Autodesk Inventor part; units mm, degrees
ref_plane "YZ Plane" through (0, 0, 0) normal (1, 0, 0) x (0, 1, 0)
ref_plane "XZ Plane" through (0, 0, 0) normal (0, 1, 0) x (-1, 0, 0)
ref_plane "XY Plane" through (0, 0, 0) normal (0, 0, 1) x (1, 0, 0)
sketch "Sketch1" plane through (0, 0, 0) normal (0, 0, 1) x (1, 0, 0)
  line L0 (-127, 177.8) -> (127, 177.8)
  line L1 (127, 177.8) -> (127, -177.8)
  line L2 (127, -177.8) -> (-127, -177.8)
  line L3 (-127, -177.8) -> (-127, 177.8)
  point P0 (0, 0)
  dimension "d0" = 254
  dimension "d1" = 127
  dimension "d2" = 355.6
  dimension "d3" = 177.8
extrude "Extrusion1" add sketch "Sketch1" along normal blind 6.35
sketch "Sketch2" plane through (0, 0, 6.35) normal (0, 0, 1) x (1, 0, 0)
  line L0 (-114.3, 165.1) -> (114.3, 165.1) construction
  line L1 (114.3, 165.1) -> (114.3, -165.1) construction
  line L2 (114.3, -165.1) -> (-114.3, -165.1) construction
  line L3 (-114.3, -165.1) -> (-114.3, 165.1) construction
  line L4 (-127, 177.8) -> (127, 177.8) construction
  line L5 (127, -177.8) -> (-127, -177.8) construction
  line L6 (-127, -177.8) -> (-127, 177.8) construction
  line L7 (127, 177.8) -> (127, -177.8) construction
  point P0 (0, 0)
  point P1 (0, 0)
  dimension "d6" = 12.7
  dimension "d7" = 12.7
  dimension "d8" = 12.7
  dimension "d9" = 12.7
hole "Hole1" at (-114.3, 165.1, 6.35) at (114.3, 165.1, 6.35) at (114.3, -165.1, 6.35) at (-114.3, -165.1, 6.35) at (0, 0, 6.35) direction (0, 0, -1) diameter 6.7564 end through all
sketch "Sketch3" plane through (0, 0, 6.35) normal (0, 0, 1) x (1, 0, 0)
  line L0 (0, 248.92) -> (0, -248.92) construction
  point P0 (0, 0)
  point P1 (0, 119.38)
  point P2 (0, -119.38)
  dimension "d17" = 238.76
  dimension "d18" = 119.38
hole "Hole2" at (0, 119.38, 6.35) at (0, -119.38, 6.35) direction (0, 0, -1) diameter 44.45 end through all
sketch "Sketch4" plane through (0, 0, 6.35) normal (0, 0, 1) x (1, 0, 0)
  line L0 (0, -248.92) -> (0, 248.92) construction
  circle A0 centre (0, 119.38) radius 22.225 construction
  circle A1 centre (0, -119.38) radius 22.225 construction
  line L1 (-177.8, 0) -> (177.8, 0) construction
  point P0 (0, 0)
  point P1 (0, 68.58)
  point P2 (0, 43.18)
  point P3 (0, -68.58)
  point P4 (0, -43.18)
  dimension "d26" = 50.8
  dimension "d27" = 25.4
  dimension "d28" = 50.8
  dimension "d29" = 25.4
hole "Hole3" at (0, 68.58, 6.35) at (0, 43.18, 6.35) at (0, -68.58, 6.35) at (0, -43.18, 6.35) direction (0, 0, -1) diameter 3.302 end through all
fillet "Fillet1" radius 12.7 4 edges at (127, -177.8, 3.175) (-127, -177.8, 3.175) (127, 177.8, 3.175) (-127, 177.8, 3.175)
chamfer "Chamfer1" distance 3.175 angle 45 2 edges at (0, -97.155, 6.35) (0, 141.605, 6.35)
sketch "Sketch6" plane through (127, -165.1, 0) normal (1, 0, 0) x (0, 0, -1)
  line L0 (-6.35, 330.2) -> (0, 330.2)
  line L1 (-6.35, 330.2) -> (-6.35, 0)
  line L2 (0, 0) -> (-6.35, 0)
  line L3 (0, 330.2) -> (0, 0)
  line L4 (-3.175, 330.2) -> (-3.175, 0) construction
  line L5 (0, 165.1) -> (-6.35, 165.1) construction
  point P0 (-3.175, 165.1)
  point P1 (-3.175, 311.15)
  point P2 (-3.175, 19.05)
  dimension "d52" = 146.05
hole "Hole5" at (127, 0, 3.175) at (127, 146.05, 3.175) at (127, -146.05, 3.175) direction (-1, 0, 0) diameter 2.6416 depth 15.24 tip angle 118
mirror "Mirror1" about plane through (0, 0, 0) normal (1, 0, 0) of "Hole5"
properties part number "J001395" material "ALUMINUM, 6061-T651"
Here's how the part is built. I have some questions about the finished solid (model axes, mm). Coordinates: 2 decimals unless noted, no trailing zeros. Write each loop counter-clockwise with the first axis right and the second up, starting at its lowest first coordinate (ties: lowest second). Pieces come first, ordered by that corner, then holes. Notation, with made-up numbers: (65.5, -23.75) -> (118.5, -23.75) arc R12 cw to (118.5, -5.75) -> close; hole circle Ø4 at (-29.75, -19). An arc over 180 degrees is marked (long way). Use a Markdown table: item, result. Add a question column.
(1) If we section it at A-A, the plane y = 119.38: Write out the boundary of the cut face in (x, z) (3 decimals).
(2) I'm going to push a flat-ended pin straight in: P1, Ø8, axis at x = 51.5, y = -67, coming from the -Z side. Where does the tip first touch, or does it pass through?
(3) We'd pull the mould along X, two halves only. Please class faces 1 (the cylindrical face through (123.38, 173.98, 3.22)), 2 (the cylindrical face through (-123.18, 174.18, 3.22)), 3 (the cylindrical face through (-111.303, 163.541, 3.131)): +X half, -X half, draft (parallel to the pull), parting line (faces both ways), or undercut.
(4) Please list where these lines run through material, in increasing order: line 1 (X direction, y = -165.1, z = 3.25); line 2 (Y direction, x = -114.3, z = 5); line 3 (Y direction, x = 112, z = 6).
Outcome:
| question | item | result |
|---|---|---|
| 1 | outline | (-127, 0) -> (-22.225, 0) -> (-22.225, 3.175) -> (-25.4, 6.35) -> (-127, 6.35) -> close; (22.225, 0) -> (127, 0) -> (127, 6.35) -> (25.4, 6.35) -> (22.225, 3.175) -> close |
| 2 | P1 | stops at z = 0 |
| 3 | face 1 | +X half |
| 3 | face 2 | -X half |
| 3 | face 3 | undercut |
| 4 | line 1 | x = -127 to -117.68, -110.92 to 110.92, 117.68 to 127 |
| 4 | line 2 | y = -177.8 to -168.48, -161.72 to 161.72, 168.48 to 177.8 |
| 4 | line 3 | y = -177.8 to -167.57, -162.63 to 162.63, 167.57 to 177.8 |
